The listing builds one solid part. Answer for the finished solid, in the listing's coordinates (mm). Face numbers are marked on the shaded views. A direction names the side the tool comes from. Give positions to 0.01 mm unless a question says otherwise; leave off trailing zeros. Order: outer loops, then holes, each group sorted by start corner. A loop starts at its lowest first (then second) coordinate and runs counter-clockwise, first axis right, second up. Notation, with made-up numbers: (54.5, 2) - (64.5, 2) arc R31 ccw to (64.5, 26) - close; hole circle Ø6 at (34, -10.75). An arc over 180 degrees is marked (long way). Answer as CSV lines item,"result". Start each with the question number.
1. Flat-ended cylindrical pins translate along their axes: pin 1 (2 mm diameter, centred on x = 3, y = -4.5, fed in from -Z); pin 2 (1.5 mm diameter, centred on x = 2.5, y = -6.5, fed in from -Z); pin 3 (1 mm diameter, centred on x = 2, y = 5, fed in from +Z); pin 4 (1.9 mm diameter, centred on x = 4.5, z = -0.5, fed in from +Y). Find the tip coordinate at first contact, or state that the pin passes through.
2. Determine the mould class of the marked faces 1, 2 and 3 for opening direction Z: +Z half, -Z half, draft (parallel to the pull), parting line (faces both ways), or undercut.
3. Section A-A on z = 0 is taken. Give the vertices of the cut face in (x, y).
4. Which of the six approach directions +Z, -Z, +X, -X, +Y, -Y give full straight-line access (tool end or side, diameter ignored) to the marked faces 4, 5 and 6?
5. Section D-D on y = 0.25 is taken. Give the vertices of the cut face in (x, z).
6. Consider line 1 along Y through (x, z) = (3.75, 0); line 2 along Z through (x, y) = (0.5, 4.5); line 3 along Y through (x, z) = (4.25, -5.5). Determine where each line is inside the solid, lowest interval first. Write a range as [from, to].
7. Section C-C on x = 1.5 is taken. Give the vertices of the cut face in (y, z), and give its area (3 significant figures).
8. Section B-B on y = 6 is taken. Give the vertices of the cut face in (x, z).
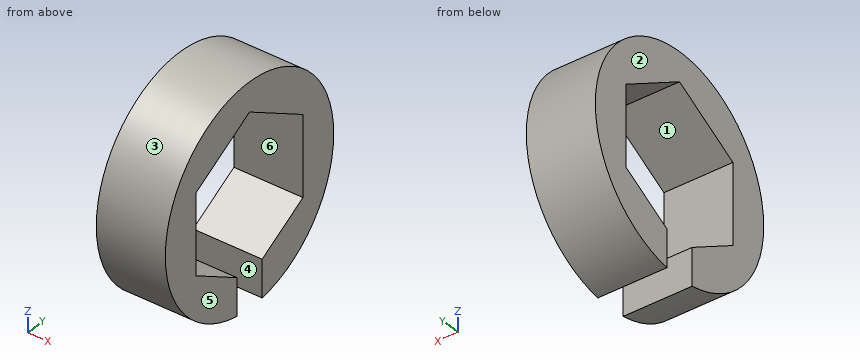
from build123d import *

# Parameters (mm, degrees)
SKETCH1_R           = 10
BOSS_EXTRUDE1_DEPTH = 6.35
SKETCH2_W           = 5.600108675
SKETCH2_H           = 3
CUT_EXTRUDE1_DEPTH  = 7.35


with BuildPart() as part:
    # Sketch1 → Boss-Extrude1 (new body)
    with BuildSketch(Plane(origin=(0, 0, 0), x_dir=(0, 0, -1), z_dir=(1, 0, 0))):
        Circle(SKETCH1_R)
        Polygon((7.332348419, 0), (3.666174209, 6.35), (-3.666174209, 6.35), (-7.332348419, 0), (-3.666174209, -6.35), (3.666174209, -6.35), align=None, mode=Mode.SUBTRACT)
    extrude(amount=BOSS_EXTRUDE1_DEPTH)

    # Sketch2 → Cut-Extrude1 (cut, through all)
    with BuildSketch(Plane(origin=(6.35, 0, 0), x_dir=(0, 0, -1), z_dir=(1, 0, 0))):
        with Locations((8.610205328, 0)):
            Rectangle(SKETCH2_W, SKETCH2_H)
    extrude(amount=-CUT_EXTRUDE1_DEPTH, mode=Mode.SUBTRACT)


solid = part.part
Checks:
1,pin 1,"stops at z = -9.37"
1,pin 2,"stops at z = -8.18"
1,pin 3,"stops at z = 8.93"
1,pin 4,"stops at y = 10"
2,face 1,"undercut"
2,face 2,"draft"
2,face 3,"parting line"
3,outline,"(0, -10) - (6.35, -10) - (6.35, -6.35) - (0, -6.35) - close; (0, 6.35) - (6.35, 6.35) - (6.35, 10) - (0, 10) - close"
4,face 4,"-Z, +X, -X"
4,face 5,"+Z, -Z, +X, +Y, -Y"
4,face 6,"+X, -X"
5,outline,"(0, 7.19) - (6.35, 7.19) - (6.35, 10) - (0, 10) - close"
6,line 1,"y = [-10, -6.35], [6.35, 10]"
6,line 2,"z = [-8.93, -4.73], [4.73, 8.93]"
6,line 3,"y = [-8.35, -3.17], [3.17, 8.35]"
7,outline,"(-6.35, -3.67) - (-6.35, 3.67) - (0, 7.33) - (6.35, 3.67) - (6.35, -3.67) - (1.5, -6.47) - (1.5, -9.89) arc R10 ccw (long way) to (-1.5, -9.89) - (-1.5, -6.47) - close"
7,area,"165 mm²"
8,outline,"(0, -8) - (6.35, -8) - (6.35, -3.87) - (0, -3.87) - close; (0, 3.87) - (6.35, 3.87) - (6.35, 8) - (0, 8) - close"
